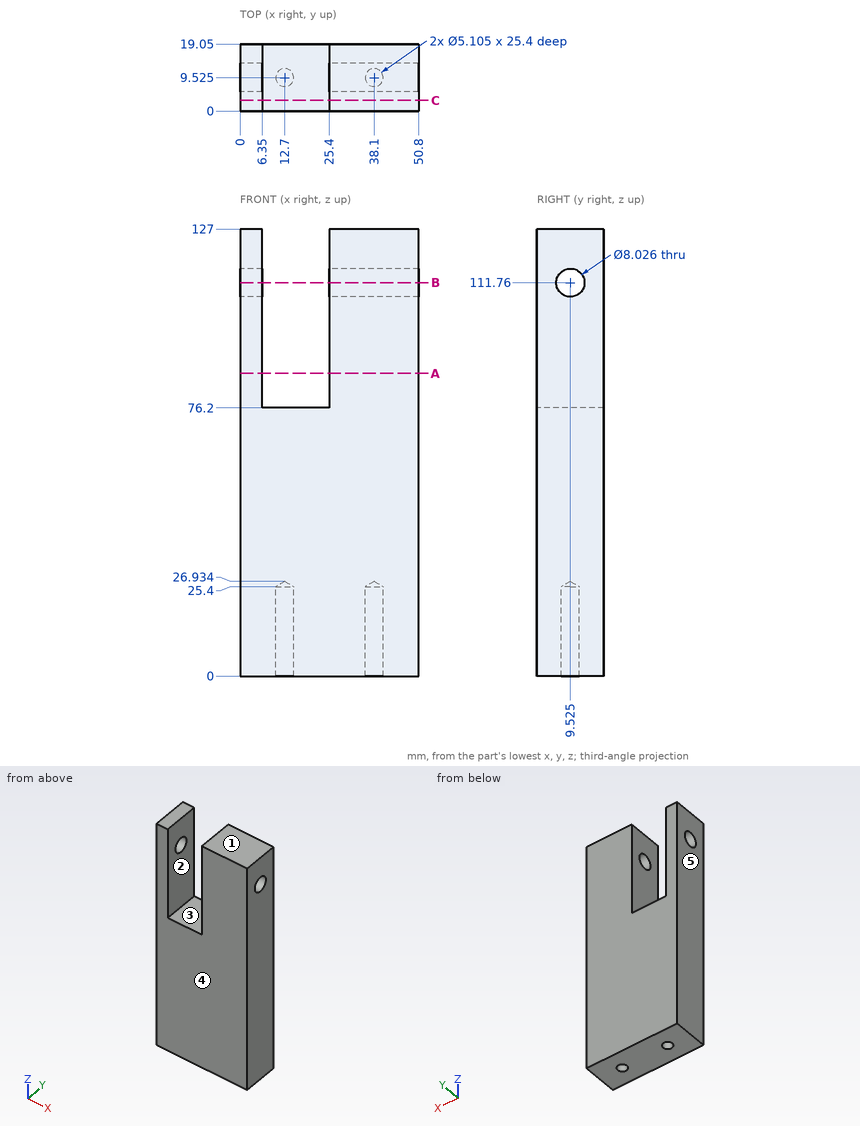
Geometry: see drawing. Coordinates: mm, zero at the bounding-box minimum. A direction names the side the tool comes from. Round coordinates to 2 decimals unless told otherwise and drop trailing zeros. Write each loop counter-clockwise with the first axis right and the second up, starting at its lowest first coordinate (ties: lowest second). Pieces come first, ordered by that corner, then holes.
Item 1: Section query A-A (z = 86). Return loops of the section in (x, y).
Item 2: Set-up query: the marked faces 1 and 2. Return all of +Z, -Z, +X, -X, +Y, -Y with unobstructed straight access to the full face (end or side cutting, diameter ignored); none if empty.
Item 3: Material intervals for L1, parallel to X at y = 5.75, z = 92; L2, parallel to Y at x = 12.7, z = 11.75; L3, parallel to Z at x = 44.5, y = 9.25, sorted ascending.
Item 4: Section query C-C (y = 3). Return loops of the section in (x, z).
Item 5: Pin query (flat end, axial travel): P1, Ø4, axis at x = 14.5, y = 8.5, coming from the +Z side; P2, Ø3, axis at x = 38.1, y = 9.525, coming from the -Z side. Return the tip coordinate at first contact, or that it passes through.
Item 6: Mould query, pull axis X, two halves, no side actions, for the marked faces 3, 4 and 5. Classes: +X half, -X half, draft (parallel to the pull), parting line (faces both ways), or undercut.
Item 7: Section query B-B (z = 111.76). Return loops of the section in (x, y), plus the area to 3 significant figures.
Completed:
1. outline: (0, 0) - (6.35, 0) - (6.35, 19.05) - (0, 19.05) - close; (25.4, 0) - (50.8, 0) - (50.8, 19.05) - (25.4, 19.05) - close
2. face 1: +Z, +X, -X, +Y, -Y
2. face 2: +Z, +Y, -Y
3. L1: x = 0 to 6.35, 25.4 to 50.8
3. L2: y = 0 to 6.97, 12.08 to 19.05
3. L3: z = 0 to 107.76, 115.76 to 127
4. outline: (0, 0) - (50.8, 0) - (50.8, 127) - (25.4, 127) - (25.4, 76.2) - (6.35, 76.2) - (6.35, 127) - (0, 127) - close
5. P1: stops at z = 76.2
5. P2: stops at z = 26.03
6. face 3: undercut
6. face 4: draft
6. face 5: -X half
7. outline: (0, 0) - (6.35, 0) - (6.35, 5.51) - (0, 5.51) - close; (0, 13.54) - (6.35, 13.54) - (6.35, 19.05) - (0, 19.05) - close; (25.4, 0) - (50.8, 0) - (50.8, 5.51) - (25.4, 5.51) - close; (25.4, 13.54) - (50.8, 13.54) - (50.8, 19.05) - (25.4, 19.05) - close
7. area: 350 mm2
